Part model, mm, in its own coordinate system. Face numbers are marked on the shaded views. A direction names the side the tool comes from. Round coordinates to 2 decimals unless told otherwise and drop trailing zeros. Loops run counter-clockwise (first coordinate to the right, second up) from the corner with the lowest first, then second, coordinate; pieces in that order, holes last. Notation, with made-up numbers: M 18,-37 L 35,-37 A30 cw 35,-2 Z; hole C 37,48.5 d4. An arc over 180 degrees is marked long. Answer as CSV lines item,"result". Start each with the question number.
Item 1: Mould opens along X. For the marked faces 1, 2 and 3 say: pulls with the +X half, pulls with the -X half, needs draft (parallel to the pull), parting line crosses it, or undercut.
Item 2: Which spindle directions (+Z, -Z, +X, -X, +Y, -Y) get a long thin tool onto all of the face, cutting with end or side? Do the marked faces 4 and 5. Say none if no direction does.
Item 3: Wall check: line 1 (Y direction, x = 5, z = 10.25); line 2 (X direction, y = 0.5, z = 5.75); line 3 (Y direction, x = 10.5, z = 1.25). Give the ranges that are in metal, low to high.
Item 4: Band-saw the part on D-D (z = 7). Give the cut face in (x, y), and give its area (3 significant figures).
Item 5: Band-saw the part on A-A (x = -0.25). Give the cut face in (y, z).
Item 6: Band-saw the part on B-B (y = 1). Give the cut face in (x, z).
Item 7: Band-saw the part on C-C (x = -6). Give the cut face in (y, z).
Item 8: Drop flat-ended pins along their axis: pin 1 Ø5 at (x, z) = (-6, 7) entering from -Y; pin 2 Ø2 at (y, z) = (3, 5.5) entering from +X. Give the stop position or say it passes through.
```python
from build123d import *

# Parameters (mm, degrees)
F1_DEPTH = 14
F2_T     = -1.5
F3_R     = 2.25
F4_DEPTH = 5
F5_R     = 0.5
F6_SIZE  = 0.5


with BuildPart() as f1:
    # F0 (on Top) → F1 (new body)
    with BuildSketch(Plane.XY):
        with BuildLine():
            ThreePointArc((-12.5, -1.5), (-11.6213203436, -3.6213203436), (-9.5, -4.5))
            Line((-9.5, -4.5), (9.5, -4.5))
            ThreePointArc((9.5, -4.5), (11.6213203436, -3.6213203436), (12.5, -1.5))
            Line((12.5, -1.5), (12.5, 1.5))
            ThreePointArc((12.5, 1.5), (11.6213203436, 3.6213203436), (9.5, 4.5))
            Line((9.5, 4.5), (-9.5, 4.5))
            ThreePointArc((-9.5, 4.5), (-11.6213203436, 3.6213203436), (-12.5, 1.5))
            Line((-12.5, 1.5), (-12.5, -1.5))
        make_face()
    extrude(amount=F1_DEPTH)

    # F2
    f2_openings = [f1.faces().sort_by_distance(p)[0] for p in [
        (0, 0, 14),
        (0, 0, 0),
    ]]
    offset(amount=F2_T, openings=f2_openings)

    # F3 (on face) → F4 (cut)
    with BuildSketch(Plane.XZ.offset(4.5)):
        with Locations((-6, 7)):
            Circle(F3_R)
        with Locations((6, 7)):
            Circle(F3_R)
    extrude(amount=-F4_DEPTH, mode=Mode.SUBTRACT)

    # F5
    f5_edges = [f1.edges().sort_by_distance(p)[0] for p in [
        (0, 4.5, 0),
        (0, -3, 0),
        (3.75, -4.5, 7),
        (-8.25, -4.5, 7),
    ]]
    fillet(f5_edges, radius=F5_R)

    # F6
    f6_edges = [f1.edges().sort_by_distance(p)[0] for p in [
        (0, -4.5, 14),
        (0, -3, 14),
    ]]
    chamfer(f6_edges, length=F6_SIZE)


solid = f1.part
```
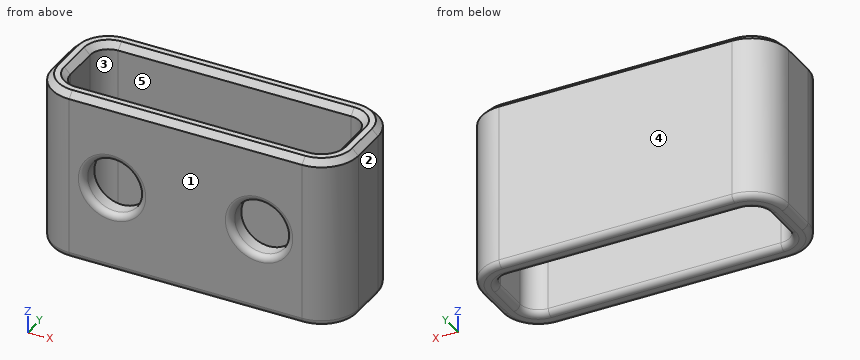
Answer block:
1,face 1,"needs draft"
1,face 2,"pulls with the +X half"
1,face 3,"undercut"
2,face 4,"+Z, -Z, +X, -X, +Y"
2,face 5,"+Z, -Z"
3,line 1,"y = -4.5 to -3, 3 to 4.5"
3,line 2,"x = -12.5 to -11, 11 to 12.5"
3,line 3,"y = -4.33 to -2.62, 2.62 to 4.33"
4,outline,"M -12.5,-1.5 A3 ccw -9.5,-4.5 L -8.75,-4.5 A0.5 ccw -8.25,-4 L -8.25,-3 L -9.5,-3 A1.5 cw -11,-1.5 L -11,1.5 A1.5 cw -9.5,3 L 9.5,3 A1.5 cw 11,1.5 L 11,-1.5 A1.5 cw 9.5,-3 L 8.25,-3 L 8.25,-4 A0.5 ccw 8.75,-4.5 L 9.5,-4.5 A3 ccw 12.5,-1.5 L 12.5,1.5 A3 ccw 9.5,4.5 L -9.5,4.5 A3 ccw -12.5,1.5 Z; M -3.75,-4 A0.5 ccw -3.25,-4.5 L 3.25,-4.5 A0.5 ccw 3.75,-4 L 3.75,-3 L -3.75,-3 Z"
4,area,"73.5 mm^2"
5,outline,"M -4.5,0.5 A0.5 ccw -4,0 L -3.5,0 A0.5 ccw -3,0.5 L -3,13.5 L -3.5,14 L -4,14 L -4.5,13.5 Z; M 3,0.5 A0.5 ccw 3.5,0 L 4,0 A0.5 ccw 4.5,0.5 L 4.5,13.5 L 4,14 L 3.5,14 L 3,13.5 Z"
6,outline,"M -12.5,0.5 A0.5 ccw -12,0 L -11.5,0 A0.5 ccw -11,0.5 L -11,13.5 L -11.5,14 L -12,14 L -12.5,13.5 Z; M 11,0.5 A0.5 ccw 11.5,0 L 12,0 A0.5 ccw 12.5,0.5 L 12.5,13.5 L 12,14 L 11.5,14 L 11,13.5 Z"
7,outline,"M -4.5,0.5 A0.5 ccw -4,0 L -3.5,0 A0.5 ccw -3,0.5 L -3,4.75 L -4,4.75 A0.5 ccw -4.5,4.25 Z; M -4.5,9.75 A0.5 ccw -4,9.25 L -3,9.25 L -3,13.5 L -3.5,14 L -4,14 L -4.5,13.5 Z; M 3,0.5 A0.5 ccw 3.5,0 L 4,0 A0.5 ccw 4.5,0.5 L 4.5,13.5 L 4,14 L 3.5,14 L 3,13.5 Z"
8,pin 1,"stops at y = -4.43"
8,pin 2,"stops at x = 12.46"
